Can you work these out from the drawing? Everything is in mm from the part's minimum corner. Round coordinates to 2 decimals unless told otherwise and drop trailing zeros. Write each loop counter-clockwise with the first axis right and the second up, starting at its lowest first coordinate (ties: lowest second). Pieces come first, ordered by that corner, then holes. Notation, with made-up numbers: (55.5, 88) -> (108.5, 88) arc R36 cw to (108.5, 123) -> close; hole circle Ø11 at (89, 51.5). An arc over 180 degrees is marked (long way). Put each result on its own line as item: value. Start each with the question number.
1. Suppose I cut it at A-A (y = 30.05). Please give me the cut outline in (x, z) (3 decimals), then the cut area to 3 significant figures.
2. I need wall thicknesses on probe 1 along Y at (x, z) = (30.05, 0.65) (3 decimals); probe 2 along Y at (x, z) = (31, 1.1); probe 3 along Y at (x, z) = (4.5, 0.4). Which ranges of each line are inside material? Lowest first, please. Write a range as from..to.
3. Suppose I cut it at B-B (z = 0.25). Count the separate pieces of the cut face and the enclosed holes in it, then the cut area to 3 significant figures.
4. Suppose I cut it at D-D (x = 54.5). Please give me the cut outline in (y, z), then the cut area to 3 significant figures.
5. For pin 1 (0.6 mm diameter, centred on y = 40.5, z = 0.5, fed in from -X); pin 2 (0.6 mm diameter, centred on x = 16.5, z = 0.5, fed in from +Y); pin 3 (0.6 mm diameter, centred on y = 15, z = 0.5, fed in from +X), each with a flat end and sliding along its axis, tell me the tip position at first contact or that it passes through.
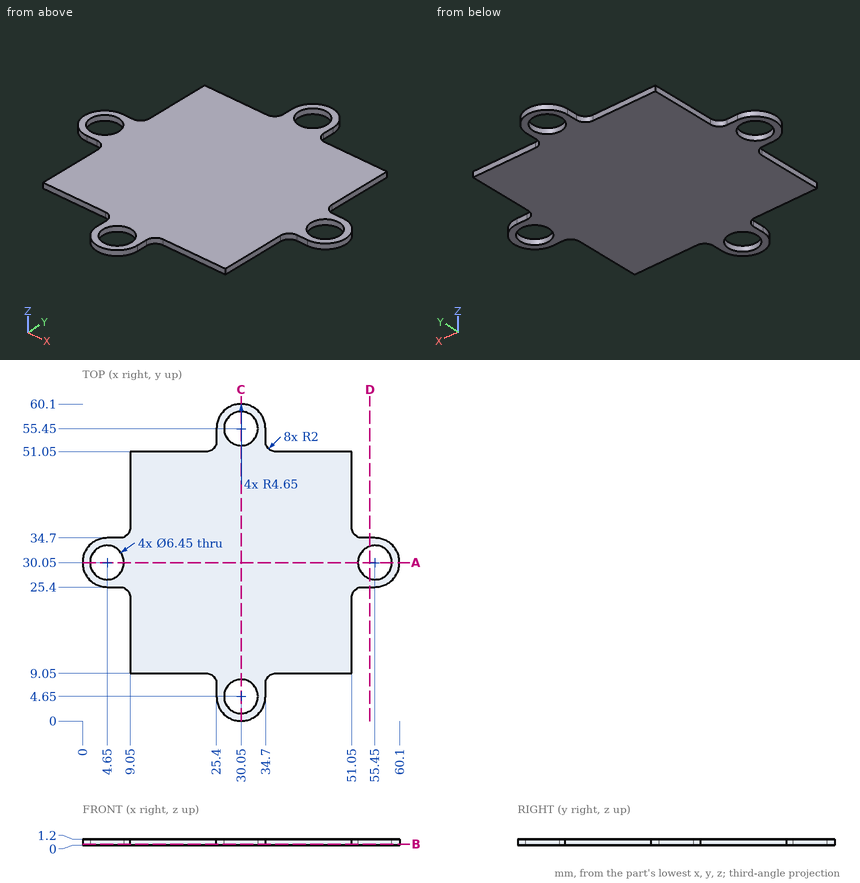
Verdict:
1. outline: (0, 0) -> (1.425, 0) -> (1.425, 1.2) -> (0, 1.2) -> close; (7.875, 0) -> (52.225, 0) -> (52.225, 1.2) -> (7.875, 1.2) -> close; (58.675, 0) -> (60.1, 0) -> (60.1, 1.2) -> (58.675, 1.2) -> close
1. area: 56.6 mm^2
2. probe 1: y = 0..1.425, 7.875..52.225, 58.675..60.1
2. probe 2: y = 0.1..1.57, 7.73..52.37, 58.53..60
2. probe 3: y = 25.4..26.83, 33.27..34.7
3. separate pieces: 1
3. enclosed holes: 4
3. area: 1,940 mm^2
4. outline: (25.4, 0) -> (26.97, 0) -> (26.97, 1.2) -> (25.4, 1.2) -> close; (33.13, 0) -> (34.7, 0) -> (34.7, 1.2) -> (33.13, 1.2) -> close
4. area: 3.76 mm^2
5. pin 1: stops at x = 9.05
5. pin 2: stops at y = 51.05
5. pin 3: stops at x = 51.05
